Part print with two shaded views. Sizes in mm from the minimum x, y, z corner. A direction names the side the tool comes from. Give positions to 0.01 mm unless a question says otherwise; leave off trailing zeros. Write each loop counter-clockwise with the first axis right and the second up, starting at its lowest first coordinate (ties: lowest second). Pieces come first, ordered by that corner, then holes. Notation, with made-up numbers: M 6,56.25 L 32,56.25 A9 cw 32,61.25 Z; hole C 40.5,47 d6. An arc over 180 degrees is marked long. Return JSON: item names as keys, results as strings. Group by question number.
Q1. Wall check: probe 1 along Z at (x, y) = (3, 7.5) (1 decimal); probe 2 along Y at (x, z) = (7.5, 36.5) (1 decimal); probe 3 along Y at (x, z) = (2, 11). Give the ranges that are in metal, low to high.
Q2. Tool access for the marked faces 1, 2 and 3: list every direction of +Z, -Z, +X, -X, +Y, -Y with a clear straight run to the whole face (end or side of a thin tool).
Q3. Band-saw the part on C-C, the plane x = 4.75. Give the cut face in (y, z) (1 decimal), then the cut area to 3 significant figures.
Q4. Flat gauge pins, fed straight in: pin 1 Ø1 at (y, z) = (7.5, 66.5) entering from +X; pin 2 Ø3 at (y, z) = (28.5, 36) entering from -X; pin 3 Ø3 at (y, z) = (7.94, 73.03) entering from -X; pin 4 Ø1.9 at (x, z) = (4, 56) entering from +Y. Where does each tip first touch, or does it go through?
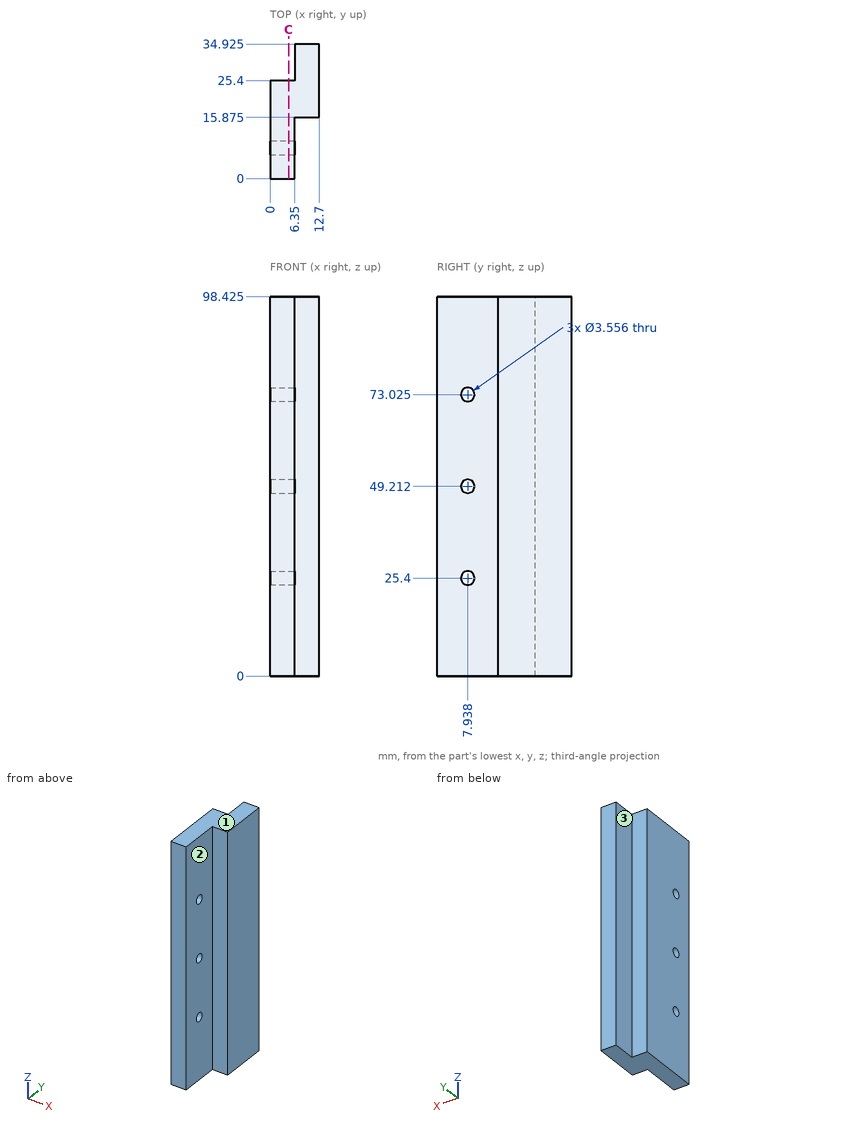
From the geometry:
{
 "1": {"probe 1": "z = 0 to 23.7, 27.1 to 47.5, 50.9 to 71.3, 74.7 to 98.4", "probe 2": "y = 15.9 to 34.9", "probe 3": "y = 0 to 25.4"},
 "2": {"face 1": "+Z, +X, -X, +Y, -Y", "face 2": "+Z, -Z, +X, -Y", "face 3": "+Z, -Z, -X, +Y"},
 "3": {"outline": "M 0,0 L 25.4,0 L 25.4,98.4 L 0,98.4 Z; hole C 7.9,25.4 d3.6; hole C 7.9,49.2 d3.6; hole C 7.9,73 d3.6", "area": "2,470 mm^2"},
 "4": {"pin 1": "stops at x = 6.35", "pin 2": "stops at x = 6.35", "pin 3": "passes through", "pin 4": "stops at y = 25.4"}
}
